Part print with two shaded views. Sizes in mm from the minimum x, y, z corner. Round coordinates to 2 decimals unless told otherwise and drop trailing zeros. Write each loop counter-clockwise with the first axis right and the second up, starting at its lowest first coordinate (ties: lowest second). Pieces come first, ordered by that corner, then holes.
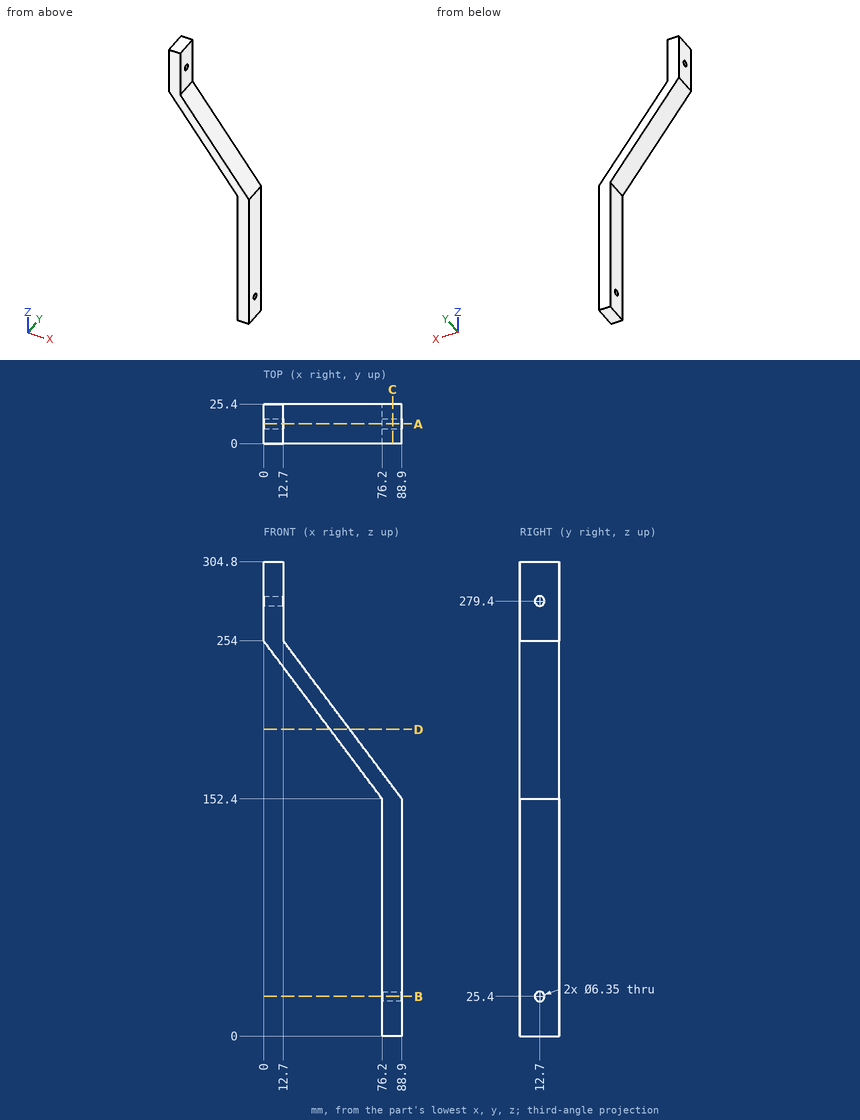
Q1. Drop flat-ended pins along their axis: pin 1 (12 mm diameter, centred on y = 14, z = 102, fed in from -X); pin 2 (1.5 mm diameter, centred on x = 58, y = 16, fed in from +Z); pin 3 (5 mm diameter, centred on y = 12.7, z = 279.4, fed in from +X); pin 4 (1 mm diameter, centred on x = 26, y = 10.5, fed in from +Z). Give the stop position or say it passes through.
Values follow:
pin 1: stops at x = 76.2
pin 2: stops at z = 194.6
pin 3: passes through
pin 4: stops at z = 236.93
Q2. Wall check: L1, parallel to Y at x = 79.5, z = 25.4 (3 decimals); L2, parallel to X at y = 13.5, z = 293; L3, parallel to X at y = 24.25, z = 35.5. Give the ranges that are in metal, low to high.
Values follow:
L1: y = 0 to 9.525, 15.875 to 25.4
L2: x = 0 to 12.7
L3: x = 76.2 to 88.9
Q3. Cut at B-B on z = 25.4. Write the cut outline in (x, y) (3 decimals), plus the area to 3 significant figures.
Values follow:
outline: (76.2, 0) - (88.9, 0) - (88.9, 9.525) - (76.2, 9.525) - close; (76.2, 15.875) - (88.9, 15.875) - (88.9, 25.4) - (76.2, 25.4) - close
area: 242 mm2
Q4. Cut at A-A on y = 12.7. Write the cut outline in (x, z) (3 decimals).
Values follow:
outline: (0, 254) - (76.2, 152.4) - (76.2, 28.575) - (88.9, 28.575) - (88.9, 152.4) - (12.7, 254) - (12.7, 276.225) - (0, 276.225) - close; (0, 282.575) - (12.7, 282.575) - (12.7, 304.8) - (0, 304.8) - close; (76.2, 0) - (88.9, 0) - (88.9, 22.225) - (76.2, 22.225) - close
Q5. Cut at C-C on x = 83. Write the cut outline in (y, z) (3 decimals).
Values follow:
outline: (0, 0) - (25.4, 0) - (25.4, 160.267) - (0, 160.267) - close; hole circle Ø6.35 at (12.7, 25.4)
Q6. Cut at D-D on z = 197. Write the cut outline in (x, y).
Values follow:
outline: (42.75, 0) - (55.45, 0) - (55.45, 25.4) - (42.75, 25.4) - close
